Check sheet for the modelled part. Datum: model origin and axes. Units: mm. Face numbers are marked on the shaded views. Coordinates: 2 decimals unless noted, no trailing zeros. Order: outer loops, then holes, each group sorted by start corner. A loop starts at its lowest first (then second) coordinate and runs counter-clockwise, first axis right, second up.
1. Cross-section at B-B (x = -40). Enter the section's corners in (y, z).
2. Gauge pin test, flat ends, axial feed: pin 1 Ø4 at (x, y) = (4.5, 48) entering from +Z; pin 2 Ø2 at (x, z) = (50, 29.54) entering from +Y. Record the tip position at first contact, or that the pin passes through.
3. Cross-section at C-C (y = 44). Enter the section's corners in (x, z), then the cut area to 3 significant figures.
4. Cross-section at A-A (y = -50). Enter the section's corners in (x, z).
5. Thickness scan on line 1 (Y direction, x = 40, z = 24.75); line 2 (X direction, y = 50.5, z = 24); line 3 (Y direction, x = -49.5, z = 32.25). Record the ranges inside material, lowest first.
6. Draft check along Y on the marked faces 1 and 2. Enter one of: released by +Y, released by -Y, zero draft, split by the parting line, or undercut.
7. Cross-section at D-D (x = 25.5). Enter the section's corners in (y, z).
```python
from build123d import *

# Parameters (mm, degrees)
F1_DEPTH  = 55
F2_W      = 90
F2_H      = 6
F3_DEPTH  = 25
F4_R      = 1.75
F5_DEPTH  = 130.001
F7_DEPTH  = 3
F9_DEPTH  = 3
F10_R     = 1.4
F11_DEPTH = 25


with BuildPart() as f1:
    # F0 (on Right) → F1 (new body, symmetric)
    with BuildSketch(Plane.YZ):
        Polygon((59, 25.4), (0, 25.4), (-59, 25.4), (-59, 35.4), (-65, 35.4), (-65, 23.4), (0, 23.4), (65, 23.4), (65, 35.4), (59, 35.4), align=None)
    extrude(amount=F1_DEPTH, both=True)

    # F2 (on face) → F3 (cut)
    with BuildSketch(Plane.XY.offset(35.4)):
        with Locations((0, 62)):
            Rectangle(F2_W, F2_H)
        with Locations((0, -62)):
            Rectangle(F2_W, F2_H)
    extrude(amount=-F3_DEPTH, mode=Mode.SUBTRACT)

    # F4 (on face) → F5 (cut, through all)
    with BuildSketch(Plane.XZ.offset(65)):
        with Locations((-50, 29.4)):
            Circle(F4_R)
        with Locations((50, 29.5409)):
            Circle(F4_R)
    extrude(amount=-F5_DEPTH, mode=Mode.SUBTRACT)

    # F6 (on face) → F7 (cut)
    with BuildSketch(Plane.XZ.offset(-59)):
        Polygon((-46.769562, 29.267323), (-48.269879, 32.131303), (-51.500317, 32.26398), (-53.230438, 29.532677), (-51.730121, 26.668697), (-48.499683, 26.53602), align=None)
        Polygon((51.730121, 26.668697), (53.230438, 29.532677), (51.500317, 32.26398), (48.269879, 32.131303), (46.769562, 29.267323), (48.499683, 26.53602), align=None)
    extrude(amount=-F7_DEPTH, mode=Mode.SUBTRACT)

    # F8 (on face) → F9 (cut)
    with BuildSketch(Plane(origin=(0, -59, 0), x_dir=(-1, 0, 0), z_dir=(0, 1, 0))):
        Polygon((-47.344236, 29.556816), (-48.685902, 31.848817), (-51.341665, 31.832901), (-52.655764, 29.524984), (-51.314098, 27.232983), (-48.658335, 27.248899), align=None)
        Polygon((51.341665, 31.832901), (48.685902, 31.848817), (47.344236, 29.556816), (48.658335, 27.248899), (51.314098, 27.232983), (52.655764, 29.524984), align=None)
    extrude(amount=-F9_DEPTH, mode=Mode.SUBTRACT)

    # F10 (on face) → F11 (cut)
    with BuildSketch(Plane.XY.offset(25.4)):
        with Locations((-40, 50)):
            Circle(F10_R)
        with Locations((40, 50)):
            Circle(F10_R)
        with Locations((-40, -50)):
            Circle(F10_R)
        with Locations((40, -50)):
            Circle(F10_R)
    extrude(amount=-F11_DEPTH, mode=Mode.SUBTRACT)


solid = f1.part
```
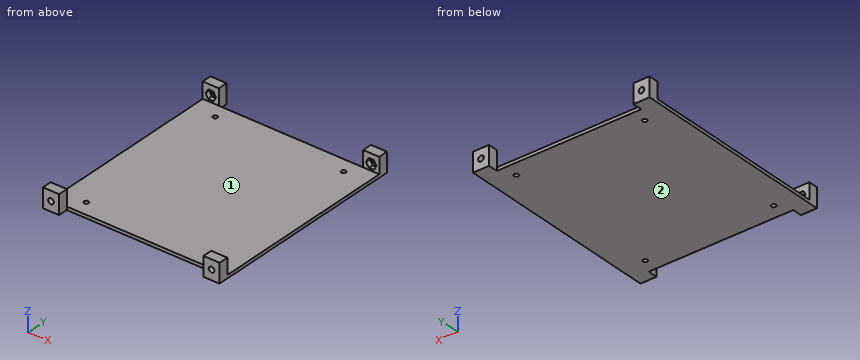
Data:
1. outline: (-59, 23.4) - (-51.4, 23.4) - (-51.4, 25.4) - (-59, 25.4) - close; (-48.6, 23.4) - (48.6, 23.4) - (48.6, 25.4) - (-48.6, 25.4) - close; (51.4, 23.4) - (59, 23.4) - (59, 25.4) - (51.4, 25.4) - close
2. pin 1: stops at z = 25.4
2. pin 2: passes through
3. outline: (-55, 23.4) - (55, 23.4) - (55, 25.4) - (-55, 25.4) - close
3. area: 220 mm2
4. outline: (-55, 23.4) - (-41.4, 23.4) - (-41.4, 25.4) - (-55, 25.4) - close; (-38.6, 23.4) - (38.6, 23.4) - (38.6, 25.4) - (-38.6, 25.4) - close; (41.4, 23.4) - (55, 23.4) - (55, 25.4) - (41.4, 25.4) - close
5. line 1: y = -59 to -51.4, -48.6 to 48.6, 51.4 to 59
5. line 2: x = -55 to -41.31, -38.69 to 38.69, 41.31 to 55
5. line 3: y = -65 to -59, 59 to 65
6. face 1: undercut
6. face 2: zero draft
7. outline: (-59, 23.4) - (59, 23.4) - (59, 25.4) - (-59, 25.4) - close
